Model file for the job. Use its own axes, mm. A direction names the side the tool comes from. Coordinates: 2 decimals unless noted, no trailing zeros. Order: outer loops, then holes, each group sorted by start corner. A loop starts at its lowest first (then second) coordinate and runs counter-clockwise, first axis right, second up. Notation, with made-up numbers: M 14.5,38 L 61.5,38 A29 cw 61.5,59 Z; hole C 45,-8 d5. An arc over 180 degrees is marked long. Return JSON: item names as keys, results as strings.
```python
from build123d import *

# Parameters (mm, degrees)
F0_R     = 7.367097
F1_DEPTH = 63.5
F2_R     = 6.35
F3_R     = 6.35
F4_R     = 3.175
F5_DEPTH = 6.35


with BuildPart() as f1:
    # F0 (on Front) → F1 (new body)
    with BuildSketch(Plane.XZ):
        Circle(F0_R)
    extrude(amount=F1_DEPTH)

    # F2
    f2_edges = [f1.edges().sort_by_distance(p)[0] for p in [
        (-7.367097, -63.5, 0),
    ]]
    fillet(f2_edges, radius=F2_R)

    # F3
    f3_edges = [f1.edges().sort_by_distance(p)[0] for p in [
        (-7.367097, 0, 0),
    ]]
    fillet(f3_edges, radius=F3_R)

    # F4 (on Front) → F5 (join, symmetric)
    with BuildSketch(Plane.XZ):
        Circle(F4_R)
    extrude(amount=F5_DEPTH, both=True)


solid = f1.part
```
Item 1: Saw through at A-A (y = -26.5). Write the cut outline in (x, z), and give its area (3 significant figures).
Check result:
{"outline": "C 0,0 d14.73", "area": "171 mm2"}
Item 2: Drop flat-ended pins along their axis: pin 1 Ø2 at (y, z) = (-27, -5) entering from -X; pin 2 Ø6 at (y, z) = (-48, 4) entering from -X; pin 3 Ø1.5 at (y, z) = (-53.5, 5.5) entering from -X. Give the stop position or say it passes through.
Check result:
{"pin 1": "stops at x = -6.19", "pin 2": "stops at x = -7.3", "pin 3": "stops at x = -5.63"}
Item 3: 3-axis set-ups, long thin cutter, end or side, ignore diameter. For faces 1 (the flat face through (0, 6.35, 0)), 2 (the cylindrical face through (-0.69, 2.94, -3.1)): which of +Z, -Z, +X, -X, +Y, -Y reach the whole face in a straight line?
Check result:
{"face 1": "+Z, -Z, +X, -X, +Y", "face 2": "+Y"}
Item 4: Wall check: line 1 (Z direction, x = -3.5, y = -53.5); line 2 (Y direction, x = -3.5, z = 0); line 3 (Z direction, x = -1, y = -2). Give the ranges that are in metal, low to high.
Check result:
{"line 1": "z = -6.48 to 6.48", "line 2": "y = -62.99 to -0.51", "line 3": "z = -5.55 to 5.55"}
